Verification items for the finished model (mm, model axes). Coordinates: 2 decimals unless noted, no trailing zeros. Order: outer loops, then holes, each group sorted by start corner. A loop starts at its lowest first (then second) coordinate and runs counter-clockwise, first axis right, second up. Notation, with made-up numbers: M 59,-1.5 L 114,-1.5 A12 cw 114,9.5 Z; hole C 12.25,20.25 d6. An arc over 180 degrees is marked long. Write item = value, one per line.
```python
from build123d import *

# Parameters (mm, degrees)
SKETCH_1_R          = 25
EXTRUDE_1_DEPTH     = 150
SKETCH_2_W          = 3.051064085
SKETCH_2_H          = 16.585271438
CUT_EXTRUDE_1_DEPTH = 6


with BuildPart() as part:
    # 草图1 → 凸台-拉伸1 (new body)
    with BuildSketch(Plane.XY):
        Circle(SKETCH_1_R)
    extrude(amount=EXTRUDE_1_DEPTH)

    # 草图2 → 切除-拉伸1 (cut)
    with BuildSketch(Plane(origin=(0, 0, 0), x_dir=(-1, 0, 0), z_dir=(0, 0, -1))):
        with Locations((5.319804046, -0.899672743)):
            Rectangle(SKETCH_2_W, SKETCH_2_H)
    extrude(amount=-CUT_EXTRUDE_1_DEPTH, mode=Mode.SUBTRACT)


solid = part.part
```
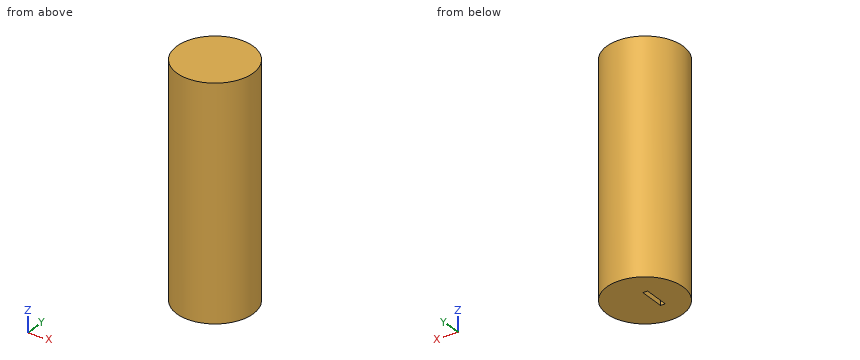
Item 1: Gauge pin test, flat ends, axial feed: pin 1 (1.5 mm diameter, centred on x = -4.5, z = 2, fed in from +Y); pin 2 (6 mm diameter, centred on x = 16, z = 71, fed in from -Y); pin 3 (1.5 mm diameter, centred on x = -5.5, y = 0, fed in from -Z). Record the tip position at first contact, or that the pin passes through.
Report:
pin_1 = 24.72
pin_2 = -21.35
pin_3 = 6
Item 2: Sectioned sample at C-C, the plane x = 7.5. Enter the section's corners in (y, z), then the cut area to 3 significant figures.
Report:
outline = M -23.85,0 L 23.85,0 L 23.85,150 L -23.85,150 Z
area = 7,150 mm^2
Item 3: Sectioned sample at A-A, the plane z = 37. Enter the section's corners in (x, y), then the cut area to 3 significant figures.
Report:
outline = C 0,0 d50
area = 1,960 mm^2
Item 4: Scan lines: L1, parallel to Y at x = 1, z = 118.5; L2, parallel to X at y = -22, z = 140.5; L3, parallel to Z at x = -5.5, y = -2. Record each from-to range of solid material in increasing order. Write a range as from..to.
Report:
L1 = -24.98..24.98
L2 = -11.87..11.87
L3 = 6..150
Item 5: Sectioned sample at B-B, the plane y = -16.5. Enter the section's corners in (x, z).
Report:
outline = M -18.78,0 L 18.78,0 L 18.78,150 L -18.78,150 Z
